Read the model definition and answer for the solid it produces. Units are mm, in the model's axes. Coordinates: 2 decimals unless noted, no trailing zeros. Write each loop counter-clockwise with the first axis right and the second up, starting at its lowest first coordinate (ties: lowest second). Pieces come first, ordered by that corner, then holes. Notation, with made-up numbers: (-5, -39.75) -> (1, -39.75) arc R23 cw to (1, -24.75) -> close; hole circle Ø9 at (27, -3.5). An arc over 180 degrees is marked (long way). Write item = value, one per line. Start each with the question number.
1) Section D-D (z = -198.5) is taken. Determine the outline of the cut face in (x, y), plus the area to 3 significant figures.
2) Section A-A (x = 10) is taken. Determine the outline of the cut face in (y, z).
3) Section B-B (y = 19.15) is taken. Count the separate pieces of the cut face and the enclosed holes in it, plus the area to 3 significant figures.
4) Find the intervals of material crossed by line 1 along X through (y, z) = (17.45, -205); line 2 along X through (y, z) = (18.6, -191); line 3 along X through (y, z) = (18.2, -208), in increasing order. Write a range as from..to.
5) A flat-ended cylindrical pin translates along its axis: pin 1 Ø5 at (x, z) = (-69.19, -220.41) entering from -Y. Find the tip coordinate at first contact, or state that the pin passes through.
6) Section C-C (x = 47.5) is taken. Determine the outline of the cut face in (y, z).
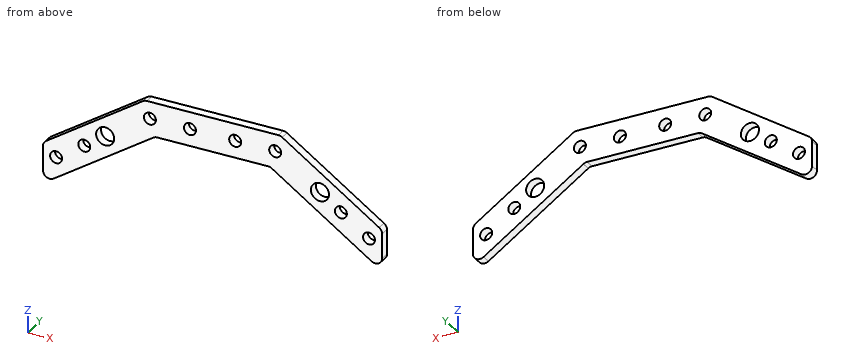
from build123d import *

# Parameters (mm, degrees)
SKETCH_1_R               = 275
SKETCH_1_R_2             = 255
EXTRUDE_1_DEPTH          = 10
EXTRUDE_2_DEPTH          = 10
SKETCH_8_R               = 2.65
SKETCH_8_R_2             = 1.65
SKETCH_8_R_3             = 2.15
CUT_EXTRUDE_1_DEPTH      = 21
SKETCH_9_OUTSIDE_W       = 707.614
SKETCH_9_OUTSIDE_H       = 707.614
CUT_EXTRUDE_2_DEPTH      = 21
SKETCH_10_W              = 150
SKETCH_10_H              = 32
CUT_EXTRUDE_3_DEPTH      = 91
SKETCH_11_R              = 275
SKETCH_11_R_2            = 255
CUT_EXTRUDE_4_DEPTH      = 11
CUT_EXTRUDE_4_DEPTH_BACK = 11
FILLET_1_R               = 3
SKETCH_13_R              = 4
CUT_EXTRUDE_6_DEPTH      = 5


with BuildPart() as part:
    # 草图1 → 凸台-拉伸1 (new body)
    with BuildSketch(Plane(origin=(0, 0, 0), x_dir=(1, 0, 0), z_dir=(0, 1, 0))):
        Circle(SKETCH_1_R)
        Circle(SKETCH_1_R_2, mode=Mode.SUBTRACT)
    extrude(amount=EXTRUDE_1_DEPTH)

    # 草图11 → 切除-拉伸4 (cut, two sides)
    with BuildSketch(Plane(origin=(0, 10, 0), x_dir=(1, 0, 0), z_dir=(0, 1, 0))) as cut_extrude_4_sk:
        Circle(SKETCH_11_R)
        Circle(SKETCH_11_R_2, mode=Mode.SUBTRACT)
    extrude(amount=CUT_EXTRUDE_4_DEPTH, mode=Mode.SUBTRACT)
    extrude(cut_extrude_4_sk.sketch, amount=-CUT_EXTRUDE_4_DEPTH_BACK, mode=Mode.SUBTRACT)


with BuildPart() as body_2:
    # 草图2 → 凸台-拉伸2 (new body)
    with BuildSketch(Plane(origin=(0, 10, 0), x_dir=(1, 0, 0), z_dir=(0, 1, 0))):
        with BuildLine():
            Line((-110.525139894, 257.262887824), (-25.423255477, 200))
            Line((-25.423255477, 200), (0, 200))
            Line((0, 200), (25.423255477, 200))
            Line((25.423255477, 200), (110.525139894, 257.262887824))
            ThreePointArc((110.525139894, 257.262887824), (197.989898732, 197.989898732), (257.262887824, 110.525139894))
            Line((257.262887824, 110.525139894), (200, 25.423255477))
            Line((200, 25.423255477), (200, 0))
            Line((200, 0), (200, -25.423255477))
            Line((200, -25.423255477), (257.262887824, -110.525139894))
            ThreePointArc((257.262887824, -110.525139894), (197.989898732, -197.989898732), (110.525139894, -257.262887824))
            Line((110.525139894, -257.262887824), (25.423255477, -200))
            Line((25.423255477, -200), (0, -200))
            Line((0, -200), (-25.423255477, -200))
            Line((-25.423255477, -200), (-110.525139894, -257.262887824))
            ThreePointArc((-110.525139894, -257.262887824), (-197.989898732, -197.989898732), (-257.262887824, -110.525139894))
            Line((-257.262887824, -110.525139894), (-200, -25.423255477))
            Line((-200, -25.423255477), (-200, 25.423255477))
            Line((-200, 25.423255477), (-257.262887824, 110.525139894))
            ThreePointArc((-257.262887824, 110.525139894), (-197.989898732, 197.989898732), (-110.525139894, 257.262887824))
        make_face()
        with BuildLine():
            Line((0, 185), (30, 185))
            Line((30, 185), (111.993839361, 240.171563565))
            ThreePointArc((111.993839361, 240.171563565), (187.383297014, 187.383297014), (240.171563565, 111.993839361))
            Line((240.171563565, 111.993839361), (185, 30))
            Line((185, 30), (185, 0))
            Line((185, 0), (185, -30))
            Line((185, -30), (240.171563565, -111.993839361))
            ThreePointArc((240.171563565, -111.993839361), (187.383297014, -187.383297014), (111.993839361, -240.171563565))
            Line((111.993839361, -240.171563565), (30, -185))
            Line((30, -185), (0, -185))
            Line((0, -185), (-30, -185))
            Line((-30, -185), (-111.993839361, -240.171563565))
            ThreePointArc((-111.993839361, -240.171563565), (-187.383297014, -187.383297014), (-240.171563565, -111.993839361))
            Line((-240.171563565, -111.993839361), (-185, -30))
            Line((-185, -30), (-185, 30))
            Line((-185, 30), (-240.171563565, 111.993839361))
            ThreePointArc((-240.171563565, 111.993839361), (-187.383297014, 187.383297014), (-111.993839361, 240.171563565))
            Line((-111.993839361, 240.171563565), (-30, 185))
            Line((-30, 185), (0, 185))
        make_face(mode=Mode.SUBTRACT)
    extrude(amount=EXTRUDE_2_DEPTH)

    # 草图8 → 切除-拉伸1 (cut, through all)
    with BuildSketch(Plane(origin=(0, 20, 0), x_dir=(1, 0, 0), z_dir=(0, 1, 0))):
        with Locations((-10, 192.5)):
            Circle(SKETCH_8_R)
        with Locations((10, 192.5)):
            Circle(SKETCH_8_R)
        with Locations((-10, -192.5)):
            Circle(SKETCH_8_R)
        with Locations((10, -192.5)):
            Circle(SKETCH_8_R)
        with Locations((192.5, 10)):
            Circle(SKETCH_8_R)
        with Locations((192.5, -10)):
            Circle(SKETCH_8_R)
        with Locations((-192.5, 10)):
            Circle(SKETCH_8_R)
        with Locations((-192.5, -10)):
            Circle(SKETCH_8_R)
        with Locations((-110.525139894, 248.223100485)):
            Circle(SKETCH_8_R_2)
        with Locations((-27.711627738, 192.5)):
            Circle(SKETCH_8_R)
        with Locations((-56.749921469, 212.03912734)):
            Circle(SKETCH_8_R)
        with Locations((-69.194904497, 220.413039057)):
            Circle(SKETCH_8_R)
        with Locations((-81.639887524, 228.786950774)):
            Circle(SKETCH_8_R)
        with Locations((-146.077022117, 230.028561882)):
            Circle(SKETCH_8_R_3)
        with Locations((-164.415519771, 217.299729706)):
            Circle(SKETCH_8_R_3)
        with Locations((-183.638937552, 201.316607082)):
            Circle(SKETCH_8_R_3)
        with Locations((-201.316607082, 183.638937552)):
            Circle(SKETCH_8_R_3)
        with Locations((-217.299729706, 164.415519771)):
            Circle(SKETCH_8_R_3)
        with Locations((-230.028561882, 146.077022117)):
            Circle(SKETCH_8_R_3)
        with Locations((-128.811575358, 240.123330241)):
            Circle(SKETCH_8_R)
        with Locations((-240.123330241, 128.811575358)):
            Circle(SKETCH_8_R)
        with Locations((-228.786950774, 81.639887524)):
            Circle(SKETCH_8_R)
        with Locations((-220.413039057, 69.194904497)):
            Circle(SKETCH_8_R)
        with Locations((-212.03912734, 56.749921469)):
            Circle(SKETCH_8_R)
        with Locations((-203.665215623, 44.304938442)):
            Circle(SKETCH_8_R)
        with Locations((-192.5, 27.711627738)):
            Circle(SKETCH_8_R)
        with Locations((-248.223100485, 110.525139894)):
            Circle(SKETCH_8_R_2)
        with Locations((192.5, 27.711627738)):
            Circle(SKETCH_8_R)
        with Locations((248.223100485, 110.525139894)):
            Circle(SKETCH_8_R_2)
        with Locations((203.665215623, 44.304938442)):
            Circle(SKETCH_8_R)
        with Locations((212.03912734, 56.749921469)):
            Circle(SKETCH_8_R)
        with Locations((220.413039057, 69.194904497)):
            Circle(SKETCH_8_R)
        with Locations((228.786950774, 81.639887524)):
            Circle(SKETCH_8_R)
        with Locations((240.123330241, 128.811575358)):
            Circle(SKETCH_8_R)
        with Locations((230.028561882, 146.077022117)):
            Circle(SKETCH_8_R_3)
        with Locations((128.811575358, 240.123330241)):
            Circle(SKETCH_8_R)
        with Locations((201.316607082, 183.638937552)):
            Circle(SKETCH_8_R_3)
        with Locations((183.638937552, 201.316607082)):
            Circle(SKETCH_8_R_3)
        with Locations((164.415519771, 217.299729706)):
            Circle(SKETCH_8_R_3)
        with Locations((146.077022117, 230.028561882)):
            Circle(SKETCH_8_R_3)
        with Locations((81.639887524, 228.786950774)):
            Circle(SKETCH_8_R)
        with Locations((69.194904497, 220.413039057)):
            Circle(SKETCH_8_R)
        with Locations((56.749921469, 212.03912734)):
            Circle(SKETCH_8_R)
        with Locations((110.525139894, 248.223100485)):
            Circle(SKETCH_8_R_2)
        with Locations((27.711627738, 192.5)):
            Circle(SKETCH_8_R)
        with Locations((217.299729706, 164.415519771)):
            Circle(SKETCH_8_R_3)
    extrude(amount=-CUT_EXTRUDE_1_DEPTH, mode=Mode.SUBTRACT)

    # 草图9 outside → 切除-拉伸2 (cut, through all)
    with BuildSketch(Plane(origin=(0, 20, 0), x_dir=(1, 0, 0), z_dir=(0, 1, 0))):
        Rectangle(SKETCH_9_OUTSIDE_W, SKETCH_9_OUTSIDE_H)
        Polygon((-75, 233.358927123), (-75, 215.279352446), (-30, 185), (30, 185), (75, 215.279352446), (75, 233.358927123), (25.423255477, 200), (-25.423255477, 200), align=None, mode=Mode.SUBTRACT)
    extrude(amount=-CUT_EXTRUDE_2_DEPTH, mode=Mode.SUBTRACT)

    # 草图10 → 切除-拉伸3 (cut, through all)
    with BuildSketch(Plane.XY.offset(-185)):
        Rectangle(SKETCH_10_W, SKETCH_10_H)
    extrude(amount=-CUT_EXTRUDE_3_DEPTH, mode=Mode.SUBTRACT)

    # 圆角1
    fillet_1_edges = [body_2.edges().sort_by_distance(p)[0] for p in [
        (-25.423255477, 18, -200),
        (25.423255477, 18, -200),
        (-75, 18, -215.279352446),
        (75, 18, -233.358927123),
        (75, 18, -215.279352446),
        (-75, 18, -233.358927123),
        (30, 18, -185),
        (-30, 18, -185),
    ]]
    fillet(fillet_1_edges, radius=FILLET_1_R)

    # 草图13 → 切除-拉伸6 (cut, through all)
    with BuildSketch(Plane.XZ.offset(-16)):
        with Locations((-47.5, -205.5)):
            Circle(SKETCH_13_R)
        with Locations((47.5, -205.5)):
            Circle(SKETCH_13_R)
    extrude(amount=-CUT_EXTRUDE_6_DEPTH, mode=Mode.SUBTRACT)


solid = body_2.part
Answer key:
q1.outline = (-50.06, 16) -> (50.06, 16) -> (50.06, 20) -> (-50.06, 20) -> close
q1.area = 401 mm^2
q2.outline = (16, -200) -> (20, -200) -> (20, -195.15) -> (16, -195.15) -> close; (16, -189.85) -> (20, -189.85) -> (20, -185) -> (16, -185) -> close
q3.separate_pieces = 1
q3.enclosed_holes = 10
q3.area = 2,250 mm^2
q4.line_1 = -59.72..-51.47, -43.53..-32.85, 32.85..43.53, 51.47..59.72
q4.line_2 = -38.92..-29.9, -25.53..-12.18, -7.82..7.82, 12.18..25.53, 29.9..38.92
q4.line_3 = -64.18..-50.62, -44.38..-37.31, 37.31..44.38, 50.62..64.18
q5.pin_1 = through
q6.outline = (16, -214.85) -> (20, -214.85) -> (20, -209.5) -> (16, -209.5) -> close; (16, -201.5) -> (20, -201.5) -> (20, -196.78) -> (16, -196.78) -> close
